Could you check a few things on this drawing? It's one solid part, dimensions in mm from its lowest x, y, z. A direction names the side the tool comes from. Round coordinates to 2 decimals unless told otherwise and drop trailing zeros. Write each loop counter-clockwise with the first axis right and the second up, starting at its lowest first coordinate (ties: lowest second). Pieces come first, ordered by that corner, then holes. Notation, with made-up numbers: (49.5, 66.5) - (89.5, 66.5) arc R32 cw to (89.5, 92.5) - close; hole circle Ø1 at (71, 15). An arc over 180 degrees is marked (long way). One line per question, with ' | ' between items. Start each with the question number.
(1) If I drill on L1, parallel to X at y = 25.5, z = 4.5; L2, parallel to Z at x = 5, y = 25, over which ranges is the centre line in solid material (lowest first)?
(2) Imagine slicing it at A-A (y = 15). Write out the boundary of the cut face in (x, z), plus the area to 3 significant figures.
(3) Will these pins go through, and if not, where does the flat tip stop? pin 1 (6.5 mm diameter, centred on y = 18, z = 21, fed in from -X); pin 2 (10.5 mm diameter, centred on y = 23.5, z = 13.5, fed in from +X); pin 3 (5 mm diameter, centred on x = 23.5, z = 5.5, fed in from +Y).
(4) Imagine slicing it at D-D (x = 30). Write out the boundary of the cut face in (y, z), plus the area to 3 significant figures.
(5) Thinking about a two-plate mould opening in Y: for the marked faces 1, 2 and 3, which applies, pulls with the +Y half, pulls with the -Y half, needs draft (parallel to the pull), parting line crosses it, or undercut?
(6) For the marked faces 4, 5 and 6, which set-ups out of +Z, -Z, +X, -X, +Y, -Y let a thin tool reach every point of the face, with its end or its side?
(7) Imagine slicing it at B-B (z = 9). Write out the boundary of the cut face in (x, y).
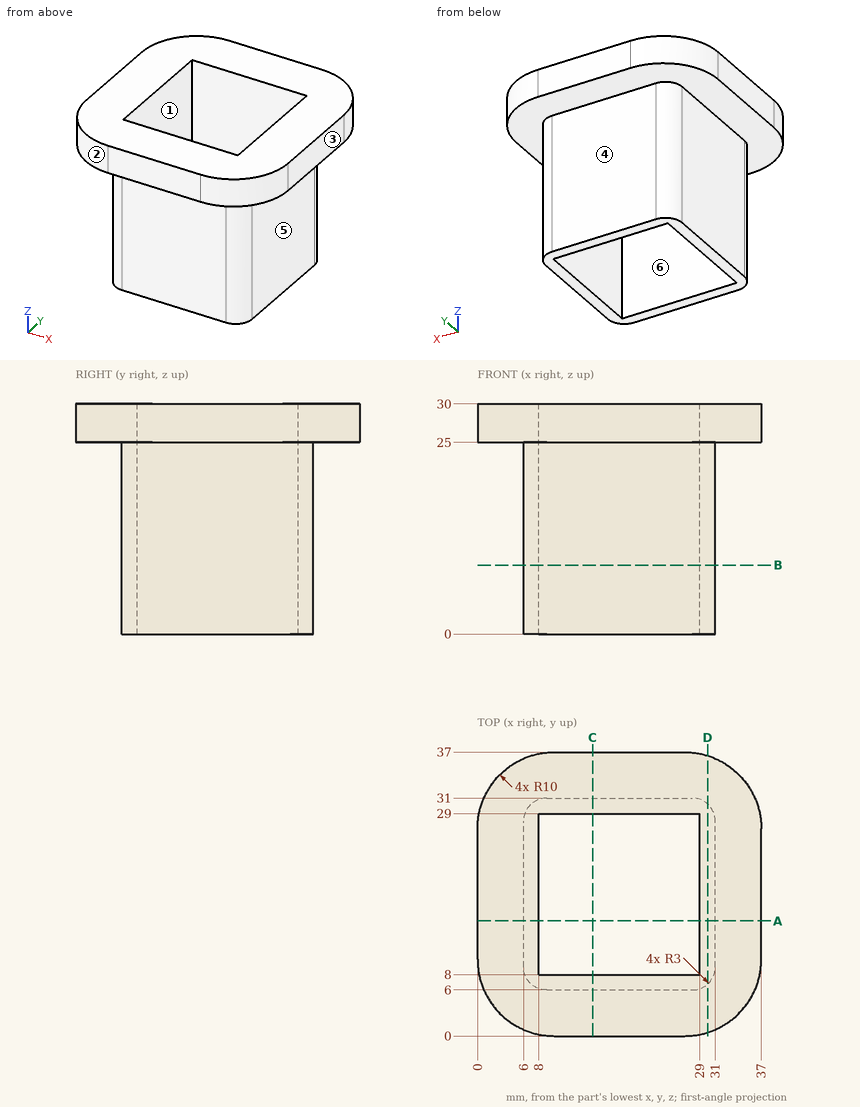
Check sheet entries:
1) L1: 6 to 8, 29 to 31 | L2: 25 to 30
2) outline: (0, 25) - (6, 25) - (6, 0) - (8, 0) - (8, 30) - (0, 30) - close; (29, 0) - (31, 0) - (31, 25) - (37, 25) - (37, 30) - (29, 30) - close | area: 180 mm^2
3) pin 1: x = 6 | pin 2: x = 31 | pin 3: y = 31
4) outline: (0.46, 25) - (6.76, 25) - (6.76, 0) - (30.24, 0) - (30.24, 25) - (36.54, 25) - (36.54, 30) - (0.46, 30) - close | area: 767 mm^2
5) face 1: undercut | face 2: pulls with the -Y half | face 3: needs draft
6) face 4: -Z, +X, -X, +Y | face 5: -Z, +X, +Y, -Y | face 6: +Z, -Z
7) outline: (6, 9) arc R3 ccw to (9, 6) - (28, 6) arc R3 ccw to (31, 9) - (31, 28) arc R3 ccw to (28, 31) - (9, 31) arc R3 ccw to (6, 28) - close; hole (8, 8) - (29, 8) - (29, 29) - (8, 29) - close
